Input: dimensioned drawing with shaded views. Units: mm. Origin: part minimum x, y, z. A direction names the side the tool comes from. Round coordinates to 2 decimals unless told otherwise and drop trailing zeros. Write each loop counter-clockwise with the first axis right and the second up, starting at its lowest first coordinate (ties: lowest second). Pieces come first, ordered by that corner, then holes. Notation, with made-up numbers: M -38,42.25 L 10,42.25 A18 cw 10,75.25 Z; hole C 39,-1.5 d2. An arc over 180 degrees is marked long. Put each result on its own line as item: value. Start each with the question number.
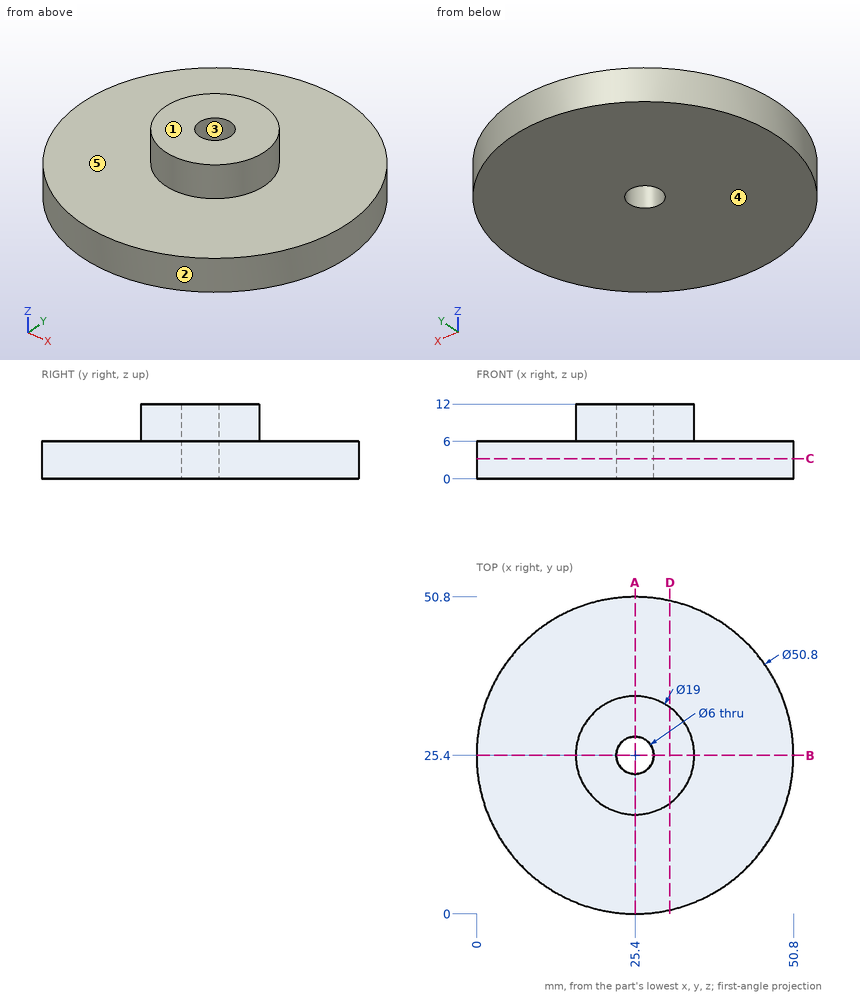
1) Section A-A, the plane x = 25.4. Output: boundary loops of the cut face in (y, z).
2) Ray query, probe 1 along Y at (x, z) = (25.4, 8.25); probe 2 along Y at (x, z) = (25.4, 4); probe 3 along Z at (x, y) = (7.5, 11). Return the intervals inside material, ascending.
3) Section D-D, the plane x = 31. Output: boundary loops of the cut face in (y, z), and give its area (3 significant figures).
4) Access query for the marked faces 4 and 5. Directions: +Z, -Z, +X, -X, +Y, -Y. A direction counts if a zero-diameter tool reaches every point of the face in a straight line with its end or side. Return the directions, or none.
5) First-contact query: pin 1 (1.5 mm diameter, centred on x = 36.5, z = 6, fed in from +Y); pin 2 (6 mm diameter, centred on x = 6, z = 3.5, fed in from +Y); pin 3 (10 mm diameter, centred on x = 11.5, y = 5.5, fed in from +Z). Flat tips, straight axial feed; report the tip coordinate or a pass-through.
6) Draft query along Y for the marked faces 1, 2 and 3. Return one class per face: +Y half, -Y half, draft (parallel to the pull), parting line (faces both ways), or undercut.
7) Section C-C, the plane z = 3.25. Output: boundary loops of the cut face in (x, y).
Solved:
1. outline: M 0,0 L 22.4,0 L 22.4,12 L 15.9,12 L 15.9,6 L 0,6 Z; M 28.4,0 L 50.8,0 L 50.8,6 L 34.9,6 L 34.9,12 L 28.4,12 Z
2. probe 1: y = 15.9 to 22.4, 28.4 to 34.9
2. probe 2: y = 0 to 22.4, 28.4 to 50.8
2. probe 3: z = 0 to 6
3. outline: M 0.63,0 L 50.17,0 L 50.17,6 L 33.07,6 L 33.07,12 L 17.73,12 L 17.73,6 L 0.63,6 Z
3. area: 389 mm2
4. face 4: -Z, +X, -X, +Y, -Y
4. face 5: +Z
5. pin 1: stops at y = 48.6
5. pin 2: stops at y = 44.8
5. pin 3: stops at z = 6
6. face 1: draft
6. face 2: parting line
6. face 3: undercut
7. outline: C 25.4,25.4 d50.8; hole C 25.4,25.4 d6
